Check sheet for the modelled part. Datum: model origin and axes. Units: mm. A direction names the side the tool comes from. Round coordinates to 2 decimals unless told otherwise and drop trailing zeros. Order: outer loops, then holes, each group sorted by start corner. A loop starts at its lowest first (then second) coordinate and runs counter-clockwise, first axis right, second up.
(1) Depth check by flat-ended pin: pin 1 (1.5 mm diameter, centred on x = 7.5, z = -2, fed in from -Y); pin 2 (2 mm diameter, centred on x = 22, z = 3, fed in from -Y); pin 3 (6 mm diameter, centred on x = 26.5, y = -4.5, fed in from -Z). Enter the tip coordinate at first touch or a pass-through.
(2) Tool access check on faces 4 (the flat face through (25, -3, 0)), 5 (the flat face through (30, 0, 0)), 6 (the flat face through (1, 0, -4)), 7 (the flat face through (1, 4, 0)), 8 (the flat face through (1, -4, 0)). Record the directions out of +Z, -Z, +X, -X, +Y, -Y that give a thin tool (end or side, any length) a straight path to the whole face; none if there is none.
(3) Mould release check, pull along X, two halves, no side actions. Record for faces 1 (the flat face through (1, 0, 4)), 2 (the flat face through (3, 2, -2)), 3 (the flat face through (0, 0, 0)): released by +X, released by -X, zero draft, split by the parting line, or undercut.
(4) Thickness scan on probe 1 along X at (y, z) = (-1, 3); probe 2 along X at (y, z) = (-1.5, 4.25); probe 3 along Z at (x, y) = (15, 0.75). Record the ranges inside material, lowest first.
(5) Sectioned sample at A-A, the plane z = 3. Enter the section's corners in (x, y).
(6) Sectioned sample at D-D, the plane y = 3.25. Enter the section's corners in (x, z).
(7) Sectioned sample at B-B, the plane y = 0. Enter the section's corners in (x, z), and give its area (3 significant figures).
```python
from build123d import *

# Parameters (mm, degrees)
SKETCH_3_W      = 8
SKETCH_3_H      = 8
EXTRUDE_1_DEPTH = 3


with BuildPart() as part:
    # 草圖1 → 旋轉1 (revolve)
    with BuildSketch(Plane.XY):
        Polygon((0, 0), (0, 2.5), (25, 2.5), (25, 6.5), (30, 6.5), (30, 0), align=None)
    revolve(axis=Axis((30, 0, 0), (-1, 0, 0)))

    # 草圖3 → 填料-伸長1 (add)
    with BuildSketch(Plane.ZY):
        Rectangle(SKETCH_3_W, SKETCH_3_H)
    extrude(amount=-EXTRUDE_1_DEPTH)


solid = part.part
```
Derived:
1. pin 1: stops at y = -2.17
1. pin 2: stops at y = -1.5
1. pin 3: stops at z = -6.32
2. face 4: none
2. face 5: +Z, -Z, +X, +Y, -Y
2. face 6: -Z, -X, +Y, -Y
2. face 7: +Z, -Z, -X, +Y
2. face 8: +Z, -Z, -X, -Y
3. face 1: zero draft
3. face 2: undercut
3. face 3: released by -X
4. probe 1: x = 0 to 3, 25 to 30
4. probe 2: x = 25 to 30
4. probe 3: z = -2.38 to 2.38
5. outline: (0, -4) - (3, -4) - (3, 4) - (0, 4) - close; (25, -5.77) - (30, -5.77) - (30, 5.77) - (25, 5.77) - close
6. outline: (0, -4) - (3, -4) - (3, 4) - (0, 4) - close; (25, -5.63) - (30, -5.63) - (30, 5.63) - (25, 5.63) - close
7. outline: (0, -4) - (3, -4) - (3, -2.5) - (25, -2.5) - (25, -6.5) - (30, -6.5) - (30, 6.5) - (25, 6.5) - (25, 2.5) - (3, 2.5) - (3, 4) - (0, 4) - close
7. area: 199 mm2
